Check sheet for the modelled part. Datum: model origin and axes. Units: mm. A direction names the side the tool comes from. Round coordinates to 2 decimals unless told otherwise and drop trailing zeros. Write each loop counter-clockwise with the first axis right and the second up, starting at its lowest first coordinate (ties: lowest second). Pieces come first, ordered by that corner, then holes.
Item 1: Section check B-B, the plane y = 9.4. Record the cut outline in (x, z).
Item 2: Section check C-C, the plane z = 2.5. Record the cut outline in (x, y).
Item 3: Material ranges on line 1 along Z through (x, y) = (-3.8, 9.4); line 2 along X through (y, z) = (8, 2.5); line 3 along Y through (x, z) = (-2.5, 5.5), recorded low to high.
Item 4: Section check A-A, the plane x = 0. Record the cut outline in (y, z), plus the area to 3 significant figures.
Item 5: Depth check by flat-ended pin: pin 1 (1.5 mm diameter, centred on x = -2.5, z = -9.5, fed in from +Y). Enter the tip coordinate at first touch or a pass-through.
Item 6: Section check D-D, the plane y = 15.5. Record the cut outline in (x, z).
Item 7: Set-up check for faces 5 (the flat face through (-2, 2, 0)), 6 (the flat face through (5, 10, 0)), 7 (the flat face through (3.5, 12, 0)): record each of +Z, -Z, +X, -X, +Y, -Y from which the full face is reachable in a straight line by a thin tool's end or side.
Item 8: Release check for a two-part mould opening along Y. For faces 1 (the cylindrical face through (-4.26, 10.008, 6.337)), 2 (the flat face through (-2.4, 3, -0.2)), 3 (the flat face through (2.3, 0, -0.2)), 4 (the cylindrical face through (-0.044, 1.521, 13.887)) record: pulls with the +Y half, pulls with the -Y half, needs draft (parallel to the pull), parting line crosses it, or undercut.
Autodesk Inventor part; units mm, degrees
ref_plane "YZ Plane" through (0, 0, 0) normal (1, 0, 0) x (0, 1, 0)
ref_plane "XZ Plane" through (0, 0, 0) normal (0, 1, 0) x (-1, 0, 0)
ref_plane "XY Plane" through (0, 0, 0) normal (0, 0, 1) x (1, 0, 0)
sketch "Sketch1" plane through (0, 0, 0) normal (0, 1, 0) x (-1, 0, 0)
  line L0 (5, -12.5) -> (-5, -12.5)
  line L1 (-5, -12.5) -> (-5, 12.5)
  line L2 (-5, 12.5) -> (5, 12.5)
  line L3 (5, 12.5) -> (5, -12.5)
  line L4 (5, -12.5) -> (-5, 12.5) construction
  line L5 (-5, -12.5) -> (5, 12.5) construction
  point P0 (0, 0)
  dimension "d0" = 10
  dimension "d1" = 25
extrude "Extrusion1" add sketch "Sketch1" along normal blind 20
sketch "Sketch2" plane through (5, 0, 12.5) normal (1, 0, 0) x (0, 0, -1)
  line L0 (0, 0) -> (25, 0)
  line L1 (0, 0) -> (0, 20)
  point P0 (12.5, 0)
  point P1 (6.9565, 9.4)
  point P2 (18.0435, 9.4)
  dimension "d11" = 9.4
  dimension "d12" = 9.4
  dimension "d13" = 11.087
  dimension "d14" = 6.9565
hole "Hole1" at (5, 9.4, 5.5435) at (5, 9.4, -5.5435) direction (-1, 0, 0) diameter 2 depth 25
sketch "Sketch3" plane through (5, 0, -12.5) normal (0, 0, -1) x (-1, 0, 0)
  line L0 (0, 0) -> (0, 20)
  line L1 (10, 0) -> (10, 20)
  line L2 (0, 20) -> (10, 20)
  line L3 (10, 20) -> (10, 0)
  line L4 (10, 0) -> (0, 0)
  line L5 (0, 0) -> (0, 20)
  point P0 (5, 0)
extrude "Extrusion2" add sketch "Sketch3" along normal blind 5
sketch "Sketch4" plane through (-5, 0, 12.5) normal (0, 0, 1) x (1, 0, 0)
  line L0 (0, 0) -> (0, 20)
  line L1 (10, 0) -> (0, 0)
  line L2 (0, 0) -> (0, 20)
  line L3 (0, 20) -> (10, 20)
  line L4 (10, 20) -> (10, 0)
  point P0 (5, 0)
extrude "Extrusion3" add sketch "Sketch4" along normal blind 5
sketch "Sketch5" plane through (0, 20, 0) normal (0, 1, 0) x (1, 0, 0)
  line L0 (0, -15.9498) -> (0, 15.9498) construction
  line L1 (3.5, -12.4498) -> (3.5, 12.4498)
  line L2 (-3.5, 12.4498) -> (-3.5, -12.4498)
  arc A0 (-3.5, -12.4498) -> (3.5, -12.4498) centre (0, -12.4498) ccw
  arc A1 (3.5, 12.4498) -> (-3.5, 12.4498) centre (0, 12.4498) ccw
  point P0 (0, 0)
  point P1 (0, 0)
  dimension "d19" = 7
extrude "Extrusion4" cut sketch "Sketch5" against normal blind 17
sketch "Sketch6" plane through (0, 3, 0) normal (0, 1, 0) x (1, 0, 0)
  line L0 (0, -13.8879) -> (0, 14.164) construction
  line L1 (2, -11.8879) -> (2, 12.164)
  line L2 (-2, 12.164) -> (-2, -11.8879)
  arc A0 (-2, -11.8879) -> (2, -11.8879) centre (0, -11.8879) ccw
  arc A1 (2, 12.164) -> (-2, 12.164) centre (0, 12.164) ccw
  point P0 (0, 0)
  point P1 (0, 0.1381)
  dimension "d22" = 4
extrude "Extrusion5" cut sketch "Sketch6" against normal blind 15
properties part number "ResonantSlider"
Values found:
1. outline: (-5, -17.5) - (5, -17.5) - (5, -6.54) - (3.5, -6.54) - (3.5, -12.45) arc R3.5 cw to (-3.5, -12.45) - (-3.5, -6.54) - (-5, -6.54) - close; (-5, -4.54) - (-3.5, -4.54) - (-3.5, 4.54) - (-5, 4.54) - close; (-5, 6.54) - (-3.5, 6.54) - (-3.5, 12.45) arc R3.5 cw to (3.5, 12.45) - (3.5, 6.54) - (5, 6.54) - (5, 17.5) - (-5, 17.5) - close; (3.5, -4.54) - (5, -4.54) - (5, 4.54) - (3.5, 4.54) - close
2. outline: (-5, 0) - (-2, 0) - (-2, 3) - (-3.5, 3) - (-3.5, 20) - (-5, 20) - close; (2, 0) - (5, 0) - (5, 20) - (3.5, 20) - (3.5, 3) - (2, 3) - close
3. line 1: z = -17.5 to -6.54, -4.54 to 4.54, 6.54 to 17.5
3. line 2: x = -5 to -3.5, 3.5 to 5
3. line 3: y = 0 to 3
4. outline: (0, -17.5) - (20, -17.5) - (20, -15.95) - (3, -15.95) - (3, -14.16) - (0, -14.16) - close; (0, 13.89) - (3, 13.89) - (3, 15.95) - (20, 15.95) - (20, 17.5) - (0, 17.5) - close
4. area: 73.6 mm2
5. pin 1: stops at y = 3
6. outline: (-5, -17.5) - (5, -17.5) - (5, 17.5) - (-5, 17.5) - close; hole (-3.5, -12.45) arc R3.5 ccw to (3.5, -12.45) - (3.5, 12.45) arc R3.5 ccw to (-3.5, 12.45) - close
7. face 5: +Y, -Y
7. face 6: +Z, -Z, +X, +Y, -Y
7. face 7: +Y
8. face 1: undercut
8. face 2: pulls with the +Y half
8. face 3: pulls with the -Y half
8. face 4: needs draft
